Can you work these out from the drawing? Everything is in mm from the part's minimum corner. Round coordinates to 2 decimals unless told otherwise and drop trailing zeros. Order: outer loops, then holes, each group sorted by start corner. A loop starts at its lowest first (then second) coordinate and runs counter-clockwise, first axis right, second up. Notation, with made-up numbers: M 20.25,-36 L 52.25,-36 A21 cw 52.25,-16 Z; hole C 3,5.25 d11. An arc over 180 degrees is marked long. Use one line per item in the form item = value. Start each with the question number.
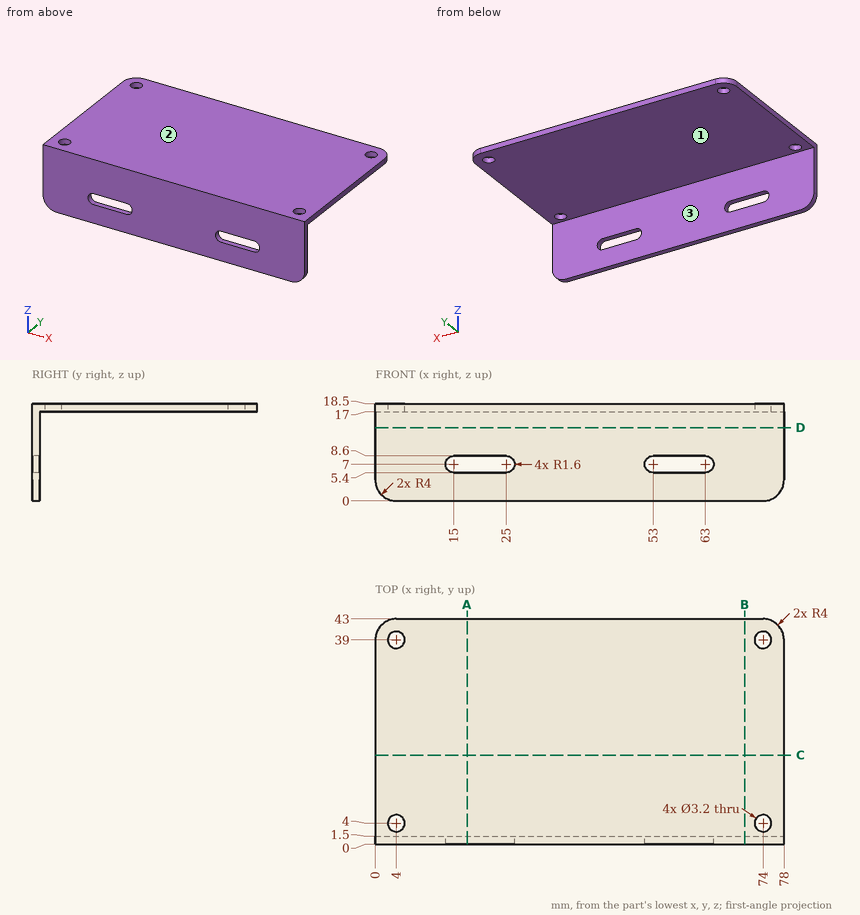
1) If we section it at B-B on x = 70.5: Write out the boundary of the cut face in (y, z), then the cut area to 3 significant figures.
2) If we mould it in two halves opening along Z, with no side actions, what happens to the marked faces 1, 2 and 3? For each: +Z half, -Z half, draft (parallel to the pull), parting line (faces both ways), or undercut.
3) Will these pins go through, and if not, where does the flat tip stop? pin 1 Ø4 at (x, y) = (40.5, 25.5) entering from -Z; pin 2 Ø10 at (x, z) = (65.5, 7) entering from +Y; pin 3 Ø2.5 at (x, y) = (4, 39) entering from -Z; pin 4 Ø6 at (x, z) = (26, 13) entering from -Y.
4) If we section it at D-D on z = 14: Write out the boundary of the cut face in (x, y), then the cut area to 3 significant figures.
5) If we section it at A-A on x = 17.5: Write out the boundary of the cut face in (y, z), then the cut area to 3 significant figures.
6) If we section it at C-C on y = 17: Write out the boundary of the cut face in (x, z), then the cut area to 3 significant figures.
7) If I drill on line 1 (Y direction, x = 74, z = 18.2); line 2 (Z direction, x = 32, y = 16.5); line 3 (Y direction, x = 69, z = 5), over which ranges is the centre line in solid material (lowest first)?
Completed:
q1.outline = M 0,0 L 1.5,0 L 1.5,17 L 43,17 L 43,18.5 L 0,18.5 Z
q1.area = 90.0 mm²
q2.face_1 = -Z half
q2.face_2 = +Z half
q2.face_3 = draft
q3.pin_1 = 17
q3.pin_2 = 1.5
q3.pin_3 = through
q3.pin_4 = 0
q4.outline = M 0,0 L 78,0 L 78,1.5 L 0,1.5 Z
q4.area = 117 mm²
q5.outline = M 0,0 L 1.5,0 L 1.5,5.4 L 0,5.4 Z; M 0,8.6 L 1.5,8.6 L 1.5,17 L 43,17 L 43,18.5 L 0,18.5 Z
q5.area = 85.2 mm²
q6.outline = M 0,17 L 78,17 L 78,18.5 L 0,18.5 Z
q6.area = 117 mm²
q7.line_1 = 0 to 2.4, 5.6 to 37.4, 40.6 to 43
q7.line_2 = 17 to 18.5
q7.line_3 = 0 to 1.5
